Source: CAD feature listing. Evaluate the final solid. Frame: model axes, mm. Face numbers are marked on the shaded views. A direction names the side the tool comes from. Coordinates: 2 decimals unless noted, no trailing zeros. Loops run counter-clockwise (first coordinate to the right, second up) from the corner with the lowest first, then second, coordinate; pieces in that order, holes last. Notation, with made-up numbers: (-10.5, -31) - (19.5, -31) arc R16 cw to (19.5, -14) - close; hole circle Ø10 at (36, 78). An arc over 180 degrees is marked (long way). Write item = value, one per line. Start each with the question number.
from build123d import *

# Parameters (mm, degrees)
SKETCH2_W           = 8
SKETCH2_H           = 18
BOSS_EXTRUDE1_DEPTH = 30
SKETCH3_R           = 2.5
CUT_EXTRUDE1_DEPTH  = 30
SKETCH5_W           = 8
SKETCH5_H           = 24
CUT_EXTRUDE2_DEPTH  = 30


with BuildPart() as part:
    # Sketch2 → Boss-Extrude1 (new body)
    with BuildSketch(Plane(origin=(0, 0, 0), x_dir=(1, 0, 0), z_dir=(0, 1, 0))):
        with Locations((4, 9)):
            Rectangle(SKETCH2_W, SKETCH2_H)
    extrude(amount=BOSS_EXTRUDE1_DEPTH)

    # Sketch3 → Cut-Extrude1 (cut)
    with BuildSketch(Plane(origin=(0, 30, 0), x_dir=(1, 0, 0), z_dir=(0, 1, 0))):
        with Locations(Location((4, 9, 0), (0, 0, 270))):
            Circle(SKETCH3_R)
    extrude(amount=-CUT_EXTRUDE1_DEPTH, mode=Mode.SUBTRACT)

    # Sketch5 → Cut-Extrude2 (cut)
    with BuildSketch(Plane(origin=(8, 0, 0), x_dir=(0, 0, -1), z_dir=(1, 0, 0))):
        with Locations((9, 15)):
            Rectangle(SKETCH5_W, SKETCH5_H)
    extrude(amount=-CUT_EXTRUDE2_DEPTH, mode=Mode.SUBTRACT)


solid = part.part
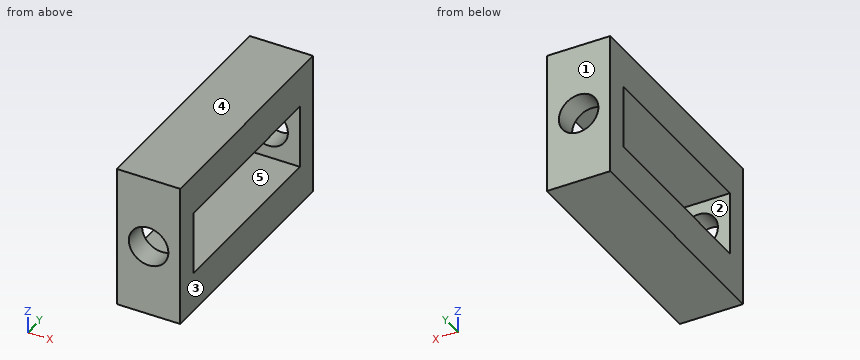
Item 1: Draft query along Y for the marked faces 1, 2 and 3. Return one class per face: released by +Y, released by -Y, zero draft, split by the parting line, or undercut.
Item 2: Cut plane C-C (x = 4). Return the cut outline in (y, z), then the cut area to 3 significant figures.
Item 3: Cut plane D-D (z = -6). Return the cut outline in (x, y).
Item 4: Reachability of the marked faces 4 and 5 from +Z, -Z, +X, -X, +Y, -Y: full face, straight path, thin tool, end or side. Return the list, or none.
Item 5: Cut plane B-B (y = 6). Return the cut outline in (x, z), then the cut area to 3 significant figures.
Item 6: Material intervals for L1, parallel to Y at x = 7.75, z = -12.5; L2, parallel to X at y = 1.25, z = -9; L3, parallel to Z at x = 6.75, y = 17.5, sorted ascending. Write a range as [from, to].
Item 7: Cut plane A-A (z = -9). Return the cut outline in (x, y).
Responses:
q1.face_1 = released by +Y
q1.face_2 = undercut
q1.face_3 = zero draft
q2.outline = (0, -18) - (30, -18) - (30, -11.5) - (27, -11.5) - (27, -13) - (3, -13) - (3, -11.5) - (0, -11.5) - close; (0, -6.5) - (3, -6.5) - (3, -5) - (27, -5) - (27, -6.5) - (30, -6.5) - (30, 0) - (0, 0) - close
q2.area = 318 mm2
q3.outline = (0, 0) - (8, 0) - (8, 3) - (0, 3) - close; (0, 27) - (8, 27) - (8, 30) - (0, 30) - close
q4.face_4 = +Z, +X, -X, +Y, -Y
q4.face_5 = +X, -X
q5.outline = (0, -18) - (8, -18) - (8, -13) - (0, -13) - close; (0, -5) - (8, -5) - (8, 0) - (0, 0) - close
q5.area = 80.0 mm2
q6.L1 = [0, 3], [27, 30]
q6.L2 = [0, 1.5], [6.5, 8]
q6.L3 = [-18, -13], [-5, 0]
q7.outline = (0, 0) - (1.5, 0) - (1.5, 3) - (0, 3) - close; (0, 27) - (1.5, 27) - (1.5, 30) - (0, 30) - close; (6.5, 0) - (8, 0) - (8, 3) - (6.5, 3) - close; (6.5, 27) - (8, 27) - (8, 30) - (6.5, 30) - close
